Build history of the part. All positions in model axes, mm. A direction names the side the tool comes from. Round coordinates to 2 decimals unless told otherwise and drop trailing zeros. Write each loop counter-clockwise with the first axis right and the second up, starting at its lowest first coordinate (ties: lowest second). Pieces come first, ordered by that corner, then holes.
Item 1: Band-saw the part on C-C, the plane z = -20.5. Write the cut outline in (x, y), then the cut area to 3 significant figures.
Item 2: Wall check: probe 1 along X at (y, z) = (0, -49.25); probe 2 along Z at (x, y) = (2.5, -11); probe 3 along Z at (x, y) = (3.5, 2.5). Give the ranges that are in metal, low to high.
Item 3: 3-axis set-ups, long thin cutter, end or side, ignore diameter. For faces 4 (the flat face through (0, -7, -1.7)), 5 (the cylindrical face through (1.393, 0.724, -58.977)), 6 (the flat face through (0, 0, -64.4)): which of +Z, -Z, +X, -X, +Y, -Y reach the whole face in a straight line?
Item 4: Band-saw the part on B-B, the plane z = -51. Write the cut outline in (x, y), then the cut area to 3 significant figures.
Item 5: Drop flat-ended pins along their axis: pin 1 Ø6.5 at (x, y) = (-12.7, 0) entering from -Z; pin 2 Ø4 at (x, y) = (-1, -7.5) entering from -Z; pin 3 Ø4 at (x, z) = (10.5, -29.5) entering from +Y. Give the stop position or say it passes through.
Item 6: Band-saw the part on D-D, the plane y = 3.5. Write the cut outline in (x, z).
Item 7: Band-saw the part on A-A, the plane x = 0. Write the cut outline in (y, z), then the cut area to 3 significant figures.
Item 8: Mould opens along Y. For faces 1 (the flat face through (-13, 0, -41.7)), 2 (the cylindrical face through (15.62, -3.47, -27.05)), 3 (the flat face through (7, 0, -51.7)) say: +Y half, -Y half, draft (parallel to the pull), parting line (faces both ways), or undercut.
```python
from build123d import *

# Parameters (mm, degrees)
SKETCH3_R      = 2
EXTRUDE1_DEPTH = 10


with BuildPart() as part:
    # Sketch2 → Revolve1 (revolve)
    with BuildSketch(Plane(origin=(0, 0, 0), x_dir=(0, 0, -1), z_dir=(1, 0, 0)), mode=Mode.PRIVATE) as revolve1_sk:
        Polygon((0, 0), (0, -6.2), (1.7, -6.2), (1.7, -16), (51.7, -16), (51.7, -6.2), (53.4, -6.2), (53.4, -1.57), (64.4, -1.57), (64.4, 0), align=None)
    revolve(revolve1_sk.sketch.rotate(Axis((0, 0, -64.4), (0, 0, 1)), 180), axis=Axis((0, 0, -64.4), (0, 0, 1)))

    # Sketch3 → Extrude1 (cut)
    with BuildSketch(Plane(origin=(0, 0, -51.7), x_dir=(-1, 0, 0), z_dir=(0, 0, -1))):
        with Locations(Location((12.7, 0, 0), (0, 0, 90))):
            Circle(SKETCH3_R)
        with Locations(Location((-12.7, 0, 0), (0, 0, 90))):
            Circle(SKETCH3_R)
    extrude(amount=-EXTRUDE1_DEPTH, mode=Mode.SUBTRACT)


solid = part.part
```
Results:
1. outline: circle Ø32 at (0, 0)
1. area: 804 mm2
2. probe 1: x = -16 to -14.7, -10.7 to 10.7, 14.7 to 16
2. probe 2: z = -51.7 to -1.7
2. probe 3: z = -53.4 to 0
3. face 4: +Z
3. face 5: -Z
3. face 6: -Z, +X, -X, +Y, -Y
4. outline: circle Ø32 at (0, 0); hole circle Ø4 at (-12.7, 0); hole circle Ø4 at (12.7, 0)
4. area: 779 mm2
5. pin 1: stops at z = -51.7
5. pin 2: stops at z = -53.4
5. pin 3: stops at y = 13.56
6. outline: (-15.61, -51.7) - (-5.12, -51.7) - (-5.12, -53.4) - (5.12, -53.4) - (5.12, -51.7) - (15.61, -51.7) - (15.61, -1.7) - (5.12, -1.7) - (5.12, 0) - (-5.12, 0) - (-5.12, -1.7) - (-15.61, -1.7) - close
7. outline: (-16, -51.7) - (-6.2, -51.7) - (-6.2, -53.4) - (-1.57, -53.4) - (-1.57, -64.4) - (1.57, -64.4) - (1.57, -53.4) - (6.2, -53.4) - (6.2, -51.7) - (16, -51.7) - (16, -1.7) - (6.2, -1.7) - (6.2, 0) - (-6.2, 0) - (-6.2, -1.7) - (-16, -1.7) - close
7. area: 1,680 mm2
8. face 1: undercut
8. face 2: parting line
8. face 3: draft
